from build123d import *

# Parameters (mm, degrees)
F0_R     = 21.725
F1_DEPTH = 25
F0_R_2   = 27.5
F2_DEPTH = 5
F3_SIZE  = 1.5


# Not quite as in the source:
# - a feature names something its author has since deleted; it is built from what else it names


with BuildPart() as f1:
    # F0 (on Top) → F1 (new body)
    with BuildSketch(Plane.XY):
        with BuildLine():
            Line((-3.2, 22.7763034753), (-3.2, 24.4414095338))
            ThreePointArc((-3.2, 24.4414095338), (-24.65, 0), (-3.2, -24.4414095338))
            Line((-3.2, -24.4414095338), (-3.2, -22.7763034753))
            Line((-3.2, -22.7763034753), (3.2, -22.7763034753))
            Line((3.2, -22.7763034753), (3.2, -24.4414095338))
            ThreePointArc((3.2, -24.4414095338), (24.65, 0), (3.2, 24.4414095338))
            Line((3.2, 24.4414095338), (3.2, 22.7763034753))
            Line((3.2, 22.7763034753), (-3.2, 22.7763034753))
        make_face()
        Circle(F0_R, mode=Mode.SUBTRACT)
    extrude(amount=F1_DEPTH)

    # F0 (on Top) → F2 (join)
    with BuildSketch(Plane.XY):
        Circle(F0_R_2)
        with BuildLine():
            ThreePointArc((-3.2, -24.4414095338), (-24.65, 0), (-3.2, 24.4414095338))
            Line((-3.2, 24.4414095338), (-3.2, 22.7763034753))
            Line((-3.2, 22.7763034753), (3.2, 22.7763034753))
            Line((3.2, 22.7763034753), (3.2, 24.4414095338))
            ThreePointArc((3.2, 24.4414095338), (24.65, 0), (3.2, -24.4414095338))
            Line((3.2, -24.4414095338), (3.2, -22.7763034753))
            Line((3.2, -22.7763034753), (-3.2, -22.7763034753))
            Line((-3.2, -22.7763034753), (-3.2, -24.4414095338))
        make_face(mode=Mode.SUBTRACT)
    extrude(amount=F2_DEPTH)

    # F3
    f3_edges = [f1.edges().sort_by_distance(p)[0] for p in [
        (-24.65, 0, 25),
        (24.65, 0, 25),
        (-21.725, 0, 0),
    ]]
    chamfer(f3_edges, length=F3_SIZE)


solid = f1.part
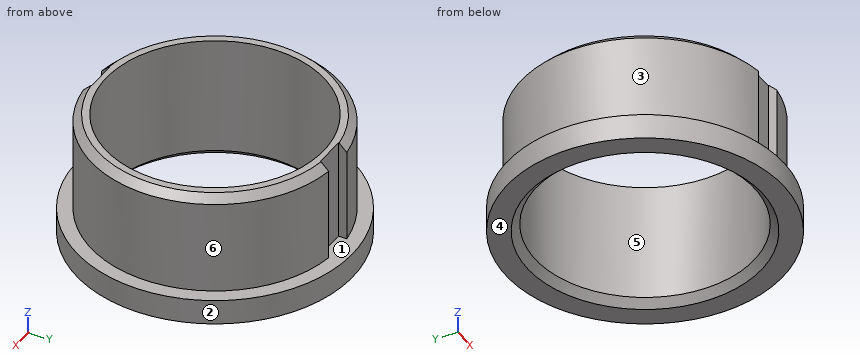
Read the model definition and answer for the solid it produces. Units are mm, in the model's axes. Face numbers are marked on the shaded views. A direction names the side the tool comes from. Coordinates: 2 decimals unless noted, no trailing zeros. Loops run counter-clockwise (first coordinate to the right, second up) from the corner with the lowest first, then second, coordinate; pieces in that order, holes last.
Q1. The part is cut by section B-B on x = 0. Write down the section's boundary in (y, z) (3 decimals).
Q2. Which of the six approach directions +Z, -Z, +X, -X, +Y, -Y give full straight-line access (tool end or side, diameter ignored) to the marked faces 1, 2 and 3?
Q3. Each of these flat-tipped pins is pushed along its axis until it touches: pin 1 Ø2 at (x, y) = (-9, -16.5) entering from +Z; pin 2 Ø1.8 at (y, z) = (23, 13.5) entering from -X; pin 3 Ø4 at (x, z) = (5, 3.5) entering from +Y; pin 4 Ø1.9 at (x, z) = (0, 13) entering from +Y. Where does it stop, or does it pass through?
Q4. The part is cut by section C-C on z = 16.25. Write down the section's boundary in (x, y) (3 decimals), and give its area (3 significant figures).
Q5. The mould has two halves that part along Y. Classify the marked faces 4, 5 and 6: +Y half, -Y half, draft (parallel to the pull), parting line (faces both ways), or undercut.
Q6. Consider probe 1 along Y at (x, z) = (0, 14.5) (3 decimals); probe 2 along X at (y, z) = (-20, 2); probe 3 along Y at (x, z) = (12, 10.25). Determine where each line is inside the solid, lowest interval first.
Q7. The part is cut by section A-A on y = 0. Write down the section's boundary in (x, z) (3 decimals).
Results below:
1. outline: (-27.5, 0) - (-23.225, 0) - (-21.725, 1.5) - (-21.725, 25) - (-22.776, 25) - (-22.776, 5) - (-27.5, 5) - close; (21.725, 1.5) - (23.225, 0) - (27.5, 0) - (27.5, 5) - (22.776, 5) - (22.776, 25) - (21.725, 25) - close
2. face 1: +Z
2. face 2: +Z, -Z
2. face 3: +Z, -X
3. pin 1: passes through
3. pin 2: stops at x = -10.92
3. pin 3: stops at y = 27.34
3. pin 4: stops at y = 22.78
4. outline: (-3.2, -24.441) - (-3.2, -22.776) - (3.2, -22.776) - (3.2, -24.441) arc R24.65 ccw to (3.2, 24.441) - (3.2, 22.776) - (-3.2, 22.776) - (-3.2, 24.441) arc R24.65 ccw to start; hole circle Ø43.45 at (0, 0)
4. area: 403 mm2
5. face 4: draft
5. face 5: undercut
5. face 6: parting line
6. probe 1: y = -22.776 to -21.725, 21.725 to 22.776
6. probe 2: x = -18.87 to -8.48, 8.48 to 18.87
6. probe 3: y = -21.53 to -18.11, 18.11 to 21.53
7. outline: (-27.5, 0) - (-23.225, 0) - (-21.725, 1.5) - (-21.725, 25) - (-23.15, 25) - (-24.65, 23.5) - (-24.65, 5) - (-27.5, 5) - close; (21.725, 1.5) - (23.225, 0) - (27.5, 0) - (27.5, 5) - (24.65, 5) - (24.65, 23.5) - (23.15, 25) - (21.725, 25) - close
